Build history of the part. All positions in model axes, mm. Round coordinates to 2 decimals unless told otherwise and drop trailing zeros. Loops run counter-clockwise (first coordinate to the right, second up) from the corner with the lowest first, then second, coordinate; pieces in that order, holes last. Notation, with made-up numbers: (-2, 68) -> (31, 68) arc R29 ccw to (31, 100) -> close; hole circle Ø5 at (6.25, -14.75). An arc over 180 degrees is marked (long way). Put each result on its own line as item: value. Start each with the question number.
Item 1: Flat gauge pins, fed straight in: pin 1 Ø1 at (x, z) = (7.5, 1.5) entering from -Y; pin 2 Ø0.6 at (y, z) = (5.5, 1) entering from +X; pin 3 Ø1 at (y, z) = (-29.5, 1) entering from +X. Where does each tip first touch, or does it go through?
Item 2: Drill centre lines: probe 1 along Y at (x, z) = (22, 1.4); probe 2 along X at (y, z) = (6, 0.95); probe 3 along X at (y, z) = (-28.5, 1.2). Where is each one in solid material? Low to high. Write a range as [from, to].
Item 3: Cut at A-A, the plane y = -45. List the corners of the cut face in (x, z), plus the area to 3 significant figures.
Item 4: Cut at D-D, the plane z = 1.1. Count the separate pieces of the cut face and the enclosed holes in it, plus the area to 3 significant figures.
Item 5: Cut at C-C, the plane x = 0.5. List the corners of the cut face in (y, z).
Item 6: Cut at B-B, the plane y = 8. List the corners of the cut face in (x, z).
```python
from build123d import *

# Parameters (mm, degrees)
SKETCH_1_R      = 1.5
SKETCH_1_W      = 2.3
SKETCH_1_H      = 5.3
SKETCH_1_W_2    = 4.3
SKETCH_1_H_2    = 8.3
EXTRUDE_1_DEPTH = 2


with BuildPart() as part:
    # 草图1 → 凸台-拉伸1 (new body)
    with BuildSketch(Plane.XY):
        Polygon((24.667061038, 17.348475873), (24.667061038, -27.701524127), (26.667061038, -27.701524127), (28.667061038, -27.701524127), (29.667061038, -55.351524127), (22.667061038, -55.351524127), (20.667061038, -55.351524127), (-8.432938962, -55.351524127), (-8.432938962, -60.451524127), (-17.332938962, -60.451524127), (-17.332938962, -14.651524127), (-17.332938962, -11.651524127), (-17.332938962, 17.348475873), align=None)
        with Locations((-14.182938962, -2.700971973)):
            Circle(SKETCH_1_R, mode=Mode.SUBTRACT)
        with Locations((21.817061038, -2.700971973)):
            Circle(SKETCH_1_R, mode=Mode.SUBTRACT)
        with Locations((24.817061038, -32.701524127)):
            Circle(SKETCH_1_R, mode=Mode.SUBTRACT)
        with Locations((-13.032938962, -48.201524127)):
            Circle(SKETCH_1_R, mode=Mode.SUBTRACT)
        with Locations((-14.182938962, -8.700971973)):
            Rectangle(SKETCH_1_W, SKETCH_1_H, mode=Mode.SUBTRACT)
        with Locations((-14.182938962, 6.299028027)):
            Rectangle(SKETCH_1_W, SKETCH_1_H, mode=Mode.SUBTRACT)
        with Locations((21.817061038, 6.299028027)):
            Rectangle(SKETCH_1_W, SKETCH_1_H, mode=Mode.SUBTRACT)
        with Locations((21.817061038, -8.700971973)):
            Rectangle(SKETCH_1_W, SKETCH_1_H, mode=Mode.SUBTRACT)
        with Locations((24.817061038, -48.201524127)):
            Rectangle(SKETCH_1_W_2, SKETCH_1_H_2, mode=Mode.SUBTRACT)
        with BuildLine():
            Line((-8.432938962, 8.949028027), (16.067061038, 8.949028027))
            Line((16.067061038, 8.949028027), (16.067061038, -37.010661405))
            add(Edge.make_bspline(
                [(11.269624681, -37.010661405), (13.852400302, -42.144100828), (16.067061038, -37.010661405)],
                knots=[0, 0, 0, 1, 1, 1], degree=2))
            Line((11.269624681, -37.010661405), (-8.432938962, 8.949028027))
        make_face(mode=Mode.SUBTRACT)
        with BuildLine():
            Line((-8.432938962, -51.551524127), (-9.251133438, -11.350971973))
            add(Edge.make_bspline(
                [(-5.718997159, -11.350971973), (-9.541336837, -6.716135438), (-9.251133438, -11.350971973)],
                knots=[0, 0, 0, 1, 1, 1], degree=2))
            Line((-5.718997159, -11.350971973), (11.269624681, -50.979915585))
            Line((11.269624681, -50.979915585), (11.514668845, -51.551524127))
            Line((11.514668845, -51.551524127), (-8.432938962, -51.551524127))
        make_face(mode=Mode.SUBTRACT)
        with Locations((-13.032938962, -54.201524127)):
            Rectangle(SKETCH_1_W, SKETCH_1_H, mode=Mode.SUBTRACT)
        with Locations((-13.032938962, -30.201524127)):
            Rectangle(SKETCH_1_W, SKETCH_1_H, mode=Mode.SUBTRACT)
    extrude(amount=EXTRUDE_1_DEPTH)


solid = part.part
```
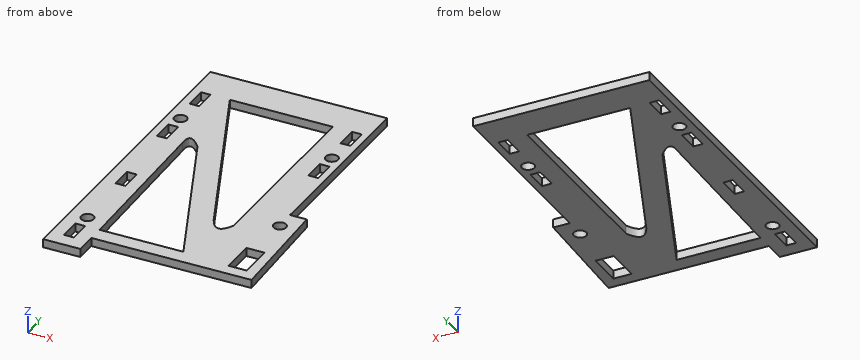
Reply:
1. pin 1: stops at y = -55.35
1. pin 2: stops at x = 24.67
1. pin 3: stops at x = 28.75
2. probe 1: y = [-55.35, -11.35], [-6.05, -4.19], [-1.21, 3.65], [8.95, 17.35]
2. probe 2: x = [-17.33, -15.33], [-13.03, -7.17], [16.07, 20.67], [22.97, 24.67]
2. probe 3: x = [-17.33, -14.18], [-11.88, -8.9], [1.63, 7.62], [16.07, 28.7]
3. outline: (-17.33, 0) -> (-8.57, 0) -> (-8.57, 2) -> (-17.33, 2) -> close; (8.71, 0) -> (22.67, 0) -> (22.67, 2) -> (8.71, 2) -> close; (26.97, 0) -> (29.29, 0) -> (29.29, 2) -> (26.97, 2) -> close
3. area: 50.1 mm^2
4. separate pieces: 1
4. enclosed holes: 13
4. area: 1,930 mm^2
5. outline: (-55.35, 0) -> (-51.55, 0) -> (-51.55, 2) -> (-55.35, 2) -> close; (-25.86, 0) -> (-11.89, 0) -> (-11.89, 2) -> (-25.86, 2) -> close; (8.95, 0) -> (17.35, 0) -> (17.35, 2) -> (8.95, 2) -> close
6. outline: (-17.33, 0) -> (-15.33, 0) -> (-15.33, 2) -> (-17.33, 2) -> close; (-13.03, 0) -> (-8.03, 0) -> (-8.03, 2) -> (-13.03, 2) -> close; (16.07, 0) -> (20.67, 0) -> (20.67, 2) -> (16.07, 2) -> close; (22.97, 0) -> (24.67, 0) -> (24.67, 2) -> (22.97, 2) -> close
